Verification items for the finished model (mm, model axes). A direction names the side the tool comes from. Give positions to 0.01 mm unless a question says otherwise; leave off trailing zeros. Order: outer loops, then holes, each group sorted by start corner. A loop starts at its lowest first (then second) coordinate and runs counter-clockwise, first axis right, second up. Notation, with made-up numbers: M 49,4.5 L 80,4.5 A22 cw 80,30.5 Z; hole C 52.25,-3 d10. An arc over 180 degrees is marked long. Answer as a JSON object with one key per item and string values.
```python
from build123d import *

# Parameters (mm, degrees)
SKETCH1_W           = 3
SKETCH1_H           = 3
BOSS_EXTRUDE1_DEPTH = 3


with BuildPart() as part:
    # Sketch1 → Boss-Extrude1 (new body)
    with BuildSketch(Plane(origin=(0, 0, 0), x_dir=(0, 0, -1), z_dir=(1, 0, 0))):
        Polygon((0, 0), (10, 0), (10, 3), (20, 3), (20, 0), (30, 0), (30, 3), (40, 3), (40, 0), (50, 0), (50, 3), (60, 3), (60, 0), (70, 0), (70, 3), (80, 3), (80, 0), (90, 0), (90, 3), (100, 3), (100, 0), (118.321595662, 0), (118.321595662, 10), (115.321595662, 10), (115.321595662, 20), (118.321595662, 20), (118.321595662, 30), (115.321595662, 30), (115.321595662, 40), (118.321595662, 40), (118.321595662, 70), (0, 90), (0, 60), (3.003699444, 60), (3.003699444, 50), (0, 50), (0, 40), (3.003699444, 40), (3.003699444, 30), (0, 30), (0, 20), (3.003699444, 20), (3.003699444, 10), (0, 10), align=None)
        with Locations((110.82, 7.5)):
            Rectangle(SKETCH1_W, SKETCH1_H, mode=Mode.SUBTRACT)
        with Locations((7.5, 7.5)):
            Rectangle(SKETCH1_W, SKETCH1_H, mode=Mode.SUBTRACT)
    extrude(amount=BOSS_EXTRUDE1_DEPTH)


solid = part.part
```
Q1. Tool access check on faces 5 (the face through (1, 7, -9)), 6 (the face through (1, 15, -115.322)), 7 (the face through (1, 3, -35)). Record the directions out of +Z, -Z, +X, -X, +Y, -Y that give a thin tool (end or side, any length) a straight path to the whole face; none if there is none.
Resolved:
{"face 5": "+X, -X", "face 6": "-Z, +X, -X", "face 7": "+X, -X, -Y"}
Q2. Section check A-A on x = 0.65. Count the separate pieces of the cut face and the enclosed holes in it, then the cut area to 3 significant figures.
Resolved:
{"separate pieces": "1", "enclosed holes": "2", "area": "9,150 mm²"}
Q3. Material ranges on L1, parallel to Z at x = 0.6, y = 19.5; L2, parallel to Y at x = 0.4, z = -96; L3, parallel to Y at x = 2.6, z = -92.5, recorded low to high.
Resolved:
{"L1": "z = -115.32 to -3", "L2": "y = 3 to 73.77", "L3": "y = 3 to 74.36"}
Q4. Release check for a two-part mould opening along Y. For faces 1 (the face through (1, 1, -30)), 2 (the face through (1, 10, -2)), 3 (the face through (1, 0, -45)), 4 (the face through (1, 30, -117)) record: +Y half, -Y half, draft (parallel to the pull), parting line (faces both ways), or undercut.
Resolved:
{"face 1": "draft", "face 2": "undercut", "face 3": "-Y half", "face 4": "undercut"}
Q5. Section check B-B on y = 55. Record the cut outline in (x, z), then the cut area to 3 significant figures.
Resolved:
{"outline": "M 0,-118.32 L 3,-118.32 L 3,-3 L 0,-3 Z", "area": "346 mm²"}
Q6. Section check C-C on z = -85.5. Record the cut outline in (x, y).
Resolved:
{"outline": "M 0,0 L 3,0 L 3,75.55 L 0,75.55 Z"}
Q7. Gauge pin test, flat ends, axial feed: pin 1 Ø1.5 at (x, y) = (2, 57.5) entering from +Z; pin 2 Ø1.5 at (x, z) = (1.5, -63.5) entering from +Y; pin 3 Ø0.9 at (x, z) = (1.5, -34) entering from -Y. Record the tip position at first contact, or that the pin passes through.
Resolved:
{"pin 1": "stops at z = -3", "pin 2": "stops at y = 79.39", "pin 3": "stops at y = 3"}
